Could you check a few things on this model? Use its own coordinates, in mm. Face numbers are marked on the shaded views. Round coordinates to 2 decimals unless told otherwise and drop trailing zeros. Write each loop counter-clockwise with the first axis right and the second up, starting at its lowest first coordinate (ties: lowest second). Pieces come first, ordered by that corner, then holes. Notation, with made-up numbers: M 68.5,-16.75 L 101.5,-16.75 A14 cw 101.5,-2.75 Z; hole C -14,-13.75 d2. An arc over 180 degrees is marked long. One line per item, written item: value. Start each with the question number.
(1) I want a section at D-D on z = -1.9. Please give me the cut outline in (x, y).
(2) I want a section at C-C on y = 17. Please give me the cut outline in (x, z) (3 decimals), and give its area (3 significant figures).
(3) I want a section at B-B on x = 0. Please give me the cut outline in (y, z), and give its area (3 significant figures).
(4) I'm going to push flat-ended pins straight in: pin 1 Ø1.5 at (y, z) = (13.5, 1) entering from +X; pin 2 Ø1 at (y, z) = (26, -1) entering from +X. Where does each tip first touch, or does it pass through?
(5) I want a section at A-A on y = 6. Please give me the cut outline in (x, z) (3 decimals), and give its area (3 significant figures).
(6) If I drill on L1, parallel to X at y = 7, z = 0; L2, parallel to Y at x = 1.75, z = 2.45; L3, parallel to Y at x = 0.5, z = 0.2, over which ranges is the centre line in solid material (lowest first)?
(7) Thinking about a two-plate mould opening in X: for the marked faces 1, 2, 3 and 4, which applies, released by +X, released by -X, zero draft, split by the parting line, or undercut?
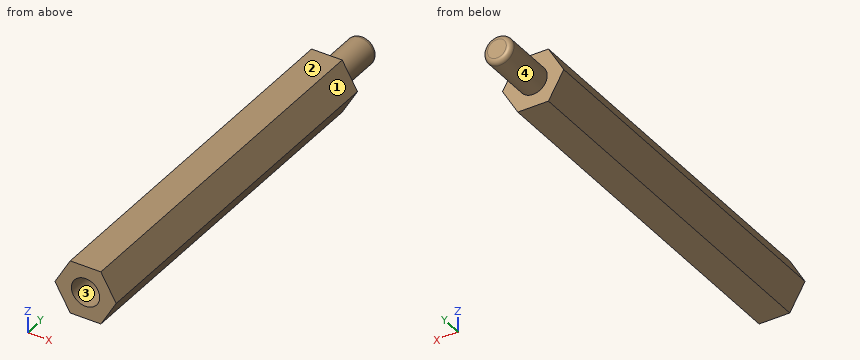
```python
from build123d import *

# Parameters (mm, degrees)
SKETCH_1_R          = 1.5
EXTRUDE_1_DEPTH     = 46
FILLET_1_R          = 0.5
SKETCH_2_R          = 1.5
EXTRUDE_2_DEPTH     = 40
SKETCH_1_2_R        = 1.5
CUT_EXTRUDE_1_DEPTH = 10


with BuildPart() as part:
    # 草图1 → 凸台-拉伸1 (new body)
    with BuildSketch(Plane(origin=(0, 0, 0), x_dir=(1, 0, 0), z_dir=(0, 1, 0))):
        with Locations(Location((0, 0, 0), (0, 0, 270))):
            Circle(SKETCH_1_R)
    extrude(amount=EXTRUDE_1_DEPTH)

    # 圆角1
    fillet_1_edges = [part.edges().sort_by_distance(p)[0] for p in [
        (0, 46, -1.5),
    ]]
    fillet(fillet_1_edges, radius=FILLET_1_R)

    # 草图2 → 凸台-拉伸2 (add)
    with BuildSketch(Plane(origin=(0, 0, 0), x_dir=(1, 0, 0), z_dir=(0, 1, 0))):
        Polygon((-1.625, 2.814582562), (-3.25, 0), (-1.625, -2.814582562), (1.625, -2.814582562), (3.25, 0), (1.625, 2.814582562), align=None)
        with Locations(Location((0, 0, 0), (0, 0, 270))):
            Circle(SKETCH_2_R, mode=Mode.SUBTRACT)
    extrude(amount=EXTRUDE_2_DEPTH)

    # 草图1<2> → 切除-拉伸1 (cut)
    with BuildSketch(Plane(origin=(0, 0, 0), x_dir=(1, 0, 0), z_dir=(0, 1, 0))):
        with Locations(Location((0, 0, 0), (0, 0, 270))):
            Circle(SKETCH_1_2_R)
    extrude(amount=CUT_EXTRUDE_1_DEPTH, mode=Mode.SUBTRACT)


solid = part.part
```
Found:
1. outline: M -2.15,0 L 2.15,0 L 2.15,40 L -2.15,40 Z
2. outline: M -3.25,0 L -1.625,-2.815 L 1.625,-2.815 L 3.25,0 L 1.625,2.815 L -1.625,2.815 Z
2. area: 27.4 mm²
3. outline: M 0,-2.81 L 40,-2.81 L 40,-1.5 L 45.5,-1.5 A0.5 ccw 46,-1 L 46,1 A0.5 ccw 45.5,1.5 L 40,1.5 L 40,2.81 L 0,2.81 L 0,1.5 L 10,1.5 L 10,-1.5 L 0,-1.5 Z
3. area: 213 mm²
4. pin 1: stops at x = 3.11
4. pin 2: stops at x = 2.96
5. outline: M -3.25,0 L -1.625,-2.815 L 1.625,-2.815 L 3.25,0 L 1.625,2.815 L -1.625,2.815 Z; hole C 0,0 d3
5. area: 20.4 mm²
6. L1: x = -3.25 to -1.5, 1.5 to 3.25
6. L2: y = 0 to 40
6. L3: y = 10 to 46
7. face 1: released by +X
7. face 2: zero draft
7. face 3: undercut
7. face 4: split by the parting line
